from build123d import *

# Parameters (mm, degrees)
SKETCH_1_R          = 7
EXTRUDE_1_DEPTH     = 150
SWEEP_2_PITCH       = 19.35483871
SWEEP_2_HEIGHT      = 150
SWEEP_2_RADIUS      = 7
SKETCH_8_R          = 3
EXTRUDE_2_DEPTH     = 5
CUT_EXTRUDE_START   = -1.5
SKETCH_9_R          = 3
CUT_EXTRUDE_1_DEPTH = 1.5


with BuildPart() as part:
    # 草圖1 → 填料-伸長1 (new body)
    with BuildSketch(Plane(origin=(0, 0, 0), x_dir=(1, 0, 0), z_dir=(0, 1, 0))):
        with Locations(Location((0, 0, 0), (0, 0, 270))):
            Circle(SKETCH_1_R)
    extrude(amount=EXTRUDE_1_DEPTH)

    # 掃出2: sweep along a helix
    with BuildLine() as sweep_2_path:
        Helix(SWEEP_2_PITCH, SWEEP_2_HEIGHT, SWEEP_2_RADIUS, center=(0, 0, 0), direction=(0, 1, 0), lefthand=True)
    # 草圖4 → 掃出2 (sweep)
    with BuildSketch(Plane(origin=(0, 0, 0), x_dir=(0, 0, -1), z_dir=(1, 0, 0))):
        Polygon((-7, 0.3), (-14.5, 0), (-7, 0), align=None)
    sweep(path=sweep_2_path.line, is_frenet=True)

    # 草圖8 → 填料-伸長2 (add)
    with BuildSketch(Plane.XZ):
        with Locations(Location((0, 0, 0), (0, 0, 90))):
            Circle(SKETCH_8_R)
    extrude(amount=EXTRUDE_2_DEPTH)

    # 草圖9 → 除料-伸長1 (cut)
    with BuildSketch(Plane.XZ.offset(5).offset(CUT_EXTRUDE_START)):
        with Locations(Location((0, 0, 0), (0, 0, 90))):
            Circle(SKETCH_9_R)
    extrude(amount=CUT_EXTRUDE_1_DEPTH, mode=Mode.SUBTRACT)


solid = part.part
CAD build for the part. Positions are in the model's coordinates, mm. A direction names the side the tool comes from. Give positions to 0.01 mm unless a question says otherwise; leave off trailing zeros. One line per question, with ' | ' between items. Start each with the question number.
1. 3-axis set-ups, long thin cutter, end or side, ignore diameter. For faces 1 (the face through (-0.9, -1.73, 2.86)), 2 (the face through (0, 150, 0)), 3 (the face through (0, -3.5, 0)): which of +Z, -Z, +X, -X, +Y, -Y reach the whole face in a straight line?
2. Saw through at A-A on z = 12. State how many separate pieces and enclosed holes the cut face has, plus the area to 3 significant figures.
3. Flat gauge pins, fed straight in: pin 1 (4 mm diameter, centred on x = 11, z = -3.5, fed in from -Y); pin 2 (8 mm diameter, centred on x = 0, z = 10.5, fed in from +Y); pin 3 (3 mm diameter, centred on x = -8, z = 7, fed in from -Y). Where does each tip first touch, or does it go through?
4. Probe L1, parallel to X at y = 59, z = -0.25; L2, parallel to Z at x = 0.5, y = 55; L3, parallel to Z at x = -3.75, y = 106.5. List the from-to ranges inside material, lowest first. Write a range as from..to.
Result sheet:
1) face 1: -Y | face 2: +Z, -Z, -X, +Y | face 3: +Z, -Z, +X, -X, -Y
2) separate pieces: 8 | enclosed holes: 0 | area: 7.98 mm^2
3) pin 1: stops at y = 13.03 | pin 2: stops at y = 150 | pin 3: stops at y = 2.19
4) L1: x = -7..7 | L2: z = -6.98..6.98 | L3: z = -5.91..5.91
